The listing builds one solid part. Answer for the finished solid, in the listing's coordinates (mm). A direction names the side the tool comes from. Round coordinates to 2 decimals unless told otherwise and drop trailing zeros. Loops run counter-clockwise (first coordinate to the right, second up) from the corner with the lowest first, then second, coordinate; pieces in that order, holes last. Notation, with made-up numbers: (43, 17) - (53, 17) arc R11 cw to (53, 34) - close; hole circle Ø10 at (30.5, -26). An arc over 180 degrees is marked (long way). One line per item, written item: value.
```python
from build123d import *

# Parameters (mm, degrees)
F0_W     = 95
F0_H     = 79
F1_DEPTH = 1
F2_W     = 95
F2_H     = 79
F2_W_2   = 66.5
F2_H_2   = 51
F3_DEPTH = 15
F4_W     = 76.5
F4_H     = 62
F4_W_2   = 66.5
F4_H_2   = 51
F5_DEPTH = 3.5
F6_W     = 56.5
F6_H     = 8.5
F6_H_2   = 10
F6_W_2   = 10
F6_H_3   = 42
F6_W_3   = 9.25
F7_DEPTH = 15
F8_R     = 1.35
F9_DEPTH = 16.001


with BuildPart() as f1:
    # F0 (on Top) → F1 (new body)
    with BuildSketch(Plane.XY):
        with Locations((47.5, 39.5)):
            Rectangle(F0_W, F0_H)
    extrude(amount=F1_DEPTH)

    # F2 (on face) → F3 (join)
    with BuildSketch(Plane.XY.offset(1)):
        with Locations((47.5, 39.5)):
            Rectangle(F2_W, F2_H)
        with Locations((47.5, 39.5)):
            Rectangle(F2_W_2, F2_H_2, mode=Mode.SUBTRACT)
    extrude(amount=F3_DEPTH)

    # F4 (on face) → F5 (cut)
    with BuildSketch(Plane.XY.offset(16)):
        with Locations((47.5, 39.5)):
            Rectangle(F4_W, F4_H)
        with Locations((47.5, 39.5)):
            Rectangle(F4_W_2, F4_H_2, mode=Mode.SUBTRACT)
    extrude(amount=-F5_DEPTH, mode=Mode.SUBTRACT)

    # F6 (on face) → F7 (cut, through all)
    with BuildSketch(Plane.XY.offset(16)):
        with Locations((47.5, 74.75)):
            Rectangle(F6_W, F6_H)
        with Locations((47.5, 65.5)):
            Rectangle(F6_W, F6_H_2)
        with Locations((14.25, 39.5)):
            Rectangle(F6_W_2, F6_H_3)
        with Locations((4.625, 39.5)):
            Rectangle(F6_W_3, F6_H_3)
        with Locations((90.375, 39.5)):
            Rectangle(F6_W_3, F6_H_3)
        with Locations((80.75, 39.5)):
            Rectangle(F6_W_2, F6_H_3)
        with Locations((47.5, 4.25)):
            Rectangle(F6_W, F6_H)
        with Locations((47.5, 13.5)):
            Rectangle(F6_W, F6_H_2)
    extrude(amount=-F7_DEPTH, mode=Mode.SUBTRACT)

    # F8 (on face) → F9 (cut, through all)
    with BuildSketch(Plane.XY.offset(16)):
        with Locations((5, 74)):
            Circle(F8_R)
        with Locations((5, 5)):
            Circle(F8_R)
        with Locations((90, 5)):
            Circle(F8_R)
        with Locations((90, 74)):
            Circle(F8_R)
    extrude(amount=-F9_DEPTH, mode=Mode.SUBTRACT)


solid = f1.part
```
1) For a pull along Y with two mould halves and no side action, classify faces 6 (the flat face through (75.75, 72, 9)), 7 (the flat face through (17, 14, 7)), 8 (the flat face through (46.8, 0, 0.8)) as released by +Y, released by -Y, zero draft, split by the parting line, or undercut.
Final values:
face 6: zero draft
face 7: undercut
face 8: released by -Y
2) A cutting plane is placed at A-A on z = 4.5. Give the vertices of the cut face in (x, y), and give its area (3 significant figures).
Final values:
outline: (0, 0) - (19.25, 0) - (19.25, 14) - (14.25, 14) - (14.25, 18.5) - (0, 18.5) - close; (0, 60.5) - (14.25, 60.5) - (14.25, 65) - (19.25, 65) - (19.25, 79) - (0, 79) - close; (75.75, 0) - (95, 0) - (95, 18.5) - (80.75, 18.5) - (80.75, 14) - (75.75, 14) - close; (75.75, 65) - (80.75, 65) - (80.75, 60.5) - (95, 60.5) - (95, 79) - (75.75, 79) - close; hole circle Ø2.7 at (5, 5); hole circle Ø2.7 at (5, 74); hole circle Ø2.7 at (90, 5); hole circle Ø2.7 at (90, 74)
area: 1,310 mm2
3) A cutting plane is placed at D-D on y = 53. Give the vertices of the cut face in (x, z), and give its area (3 significant figures).
Final values:
outline: (0, 0) - (95, 0) - (95, 1) - (0, 1) - close
area: 95.0 mm2
4) For faces 1 (the flat face through (87, 72, 16)), 2 (the flat face through (13, 12, 12.5)), 3 (the flat face through (88, 18.5, 9)), 4 (the flat face through (75.75, 7, 9)), 5 (the flat face through (95, 38.9, 0.8)), determine the directions among +Z, -Z, +X, -X, +Y, -Y from which every point of the face is accessible in a straight line to the end or side of a thin tool.
Final values:
face 1: +Z, +X, -X, +Y, -Y
face 2: +Z
face 3: +Z, +X, -X
face 4: +Z, +Y, -Y
face 5: +Z, -Z, +X, +Y, -Y
5) A cutting plane is placed at B-B on x = 90. Give the vertices of the cut face in (y, z), and give its area (3 significant figures).
Final values:
outline: (0, 0) - (3.65, 0) - (3.65, 16) - (0, 16) - close; (6.35, 0) - (72.65, 0) - (72.65, 16) - (60.5, 16) - (60.5, 1) - (18.5, 1) - (18.5, 16) - (6.35, 16) - close; (75.35, 0) - (79, 0) - (79, 16) - (75.35, 16) - close
area: 548 mm2
6) A cutting plane is placed at C-C on y = 5. Give the vertices of the cut face in (x, z), and give its area (3 significant figures).
Final values:
outline: (0, 0) - (3.65, 0) - (3.65, 16) - (0, 16) - close; (6.35, 0) - (88.65, 0) - (88.65, 16) - (75.75, 16) - (75.75, 1) - (19.25, 1) - (19.25, 16) - (6.35, 16) - close; (91.35, 0) - (95, 0) - (95, 16) - (91.35, 16) - close
area: 586 mm2
7) Each of these flat-tipped pins is pushed along its axis until it touches: pin 1 Ø2 at (x, y) = (37.5, 37) entering from +Z; pin 2 Ø2 at (x, y) = (5, 5) entering from +Z; pin 3 Ø3 at (x, y) = (81.5, 15) entering from +Z. Where does it stop, or does it pass through?
Final values:
pin 1: z = 1
pin 2: through
pin 3: z = 12.5
8) Consider L1, parallel to X at y = 74, z = 8.5; L2, parallel to Y at x = 90, z = 7.5; L3, parallel to Y at x = 77.5, z = 12.25. Determine where each line is inside the solid, lowest interval first.
Final values:
L1: 0 to 3.65, 6.35 to 19.25, 75.75 to 88.65, 91.35 to 95
L2: 0 to 3.65, 6.35 to 18.5, 60.5 to 72.65, 75.35 to 79
L3: 0 to 14, 65 to 79
